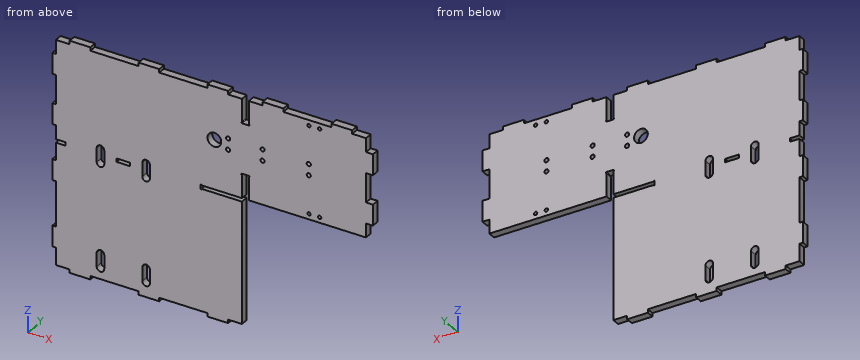
from build123d import *

# Parameters (mm, degrees)
BODY_DELETE_KEEP_START         = -69.85
BODY_DELETE_KEEP_1_OUTLINE_W   = 12.7
BODY_DELETE_KEEP_1_OUTLINE_H   = 3.175
BODY_DELETE_KEEP_1_OUTLINE_R   = 1.905
BODY_DELETE_KEEP_1_OUTLINE_R_2 = 6.35
BODY_DELETE_KEEP_1_OUTLINE_R_3 = 1.5367
BODY_DELETE_KEEP_1_DEPTH       = 6.985
SKETCH1_R                      = 0.635
CUT_EXTRUDE1_DEPTH             = 257.935529511


# Read off the part's stored shape, not the designer's step: Body-Delete/Keep 1
with BuildPart() as part:
    # Body-Delete/Keep 1 outline → Body-Delete/Keep 1 (new body)
    with BuildSketch(Plane(origin=(0, 0, 0), x_dir=(1, 0, 0), z_dir=(0, 1, 0)).offset(BODY_DELETE_KEEP_START)):
        Polygon((90.075, -13.335), (90.075, 13.335), (96.425, 13.335), (96.425, 32.385), (90.075, 32.385), (90.075, 45.085), (-17.875, 45.085), (-17.875, 22.86), (-24.225, 22.86), (-24.225, 45.085), (-62.325, 45.085), (-62.325, 48.26), (-24.225, 48.26), (-24.225, 159.385), (-36.925, 159.385), (-36.925, 162.56), (-55.975, 162.56), (-55.975, 159.385), (-100.425, 159.385), (-100.425, 162.56), (-119.475, 162.56), (-119.475, 159.385), (-163.925, 159.385), (-163.925, 162.56), (-182.975, 162.56), (-182.975, 159.385), (-195.675, 159.385), (-195.675, 143.51), (-198.85, 143.51), (-198.85, 124.46), (-195.675, 124.46), (-195.675, 83.185), (-198.85, 83.185), (-198.85, 64.135), (-195.675, 64.135), (-195.675, 48.26), (-186.785, 48.26), (-186.785, 45.085), (-195.675, 45.085), (-195.675, 32.385), (-198.85, 32.385), (-198.85, 13.335), (-195.675, 13.335), (-195.675, -13.335), (-198.85, -13.335), (-198.85, -32.385), (-195.675, -32.385), (-195.675, -45.085), (-182.975, -45.085), (-182.975, -48.26), (-163.925, -48.26), (-163.925, -45.085), (-119.475, -45.085), (-119.475, -48.26), (-100.425, -48.26), (-100.425, -45.085), (-55.975, -45.085), (-55.975, -48.26), (-36.925, -48.26), (-36.925, -45.085), (-24.225, -45.085), (-24.225, -22.86), (-17.875, -22.86), (-17.875, -45.085), (-5.175, -45.085), (-5.175, -48.26), (13.875, -48.26), (13.875, -45.085), (58.325, -45.085), (58.325, -48.26), (77.375, -48.26), (77.375, -45.085), (90.075, -45.085), (90.075, -32.385), (96.425, -32.385), (96.425, -13.335), align=None)
        with BuildLine():
            Line((-151.0668, 54.1), (-151.0668, 41.4))
            ThreePointArc((-151.0668, 41.4), (-154.5593, 37.9075), (-158.0518, 41.4))
            Line((-158.0518, 41.4), (-158.0518, 54.1))
            ThreePointArc((-158.0518, 54.1), (-154.5593, 57.5925), (-151.0668, 54.1))
        make_face(mode=Mode.SUBTRACT)
        with Locations((-133.5593, 46.6725)):
            Rectangle(BODY_DELETE_KEEP_1_OUTLINE_W, BODY_DELETE_KEEP_1_OUTLINE_H, mode=Mode.SUBTRACT)
        with BuildLine():
            Line((-109.0668, 54.1), (-109.0668, 41.4))
            ThreePointArc((-109.0668, 41.4), (-112.5593, 37.9075), (-116.0518, 41.4))
            Line((-116.0518, 41.4), (-116.0518, 54.1))
            ThreePointArc((-116.0518, 54.1), (-112.5593, 57.5925), (-109.0668, 54.1))
        make_face(mode=Mode.SUBTRACT)
        with Locations((-36.925, -5.08)):
            Circle(BODY_DELETE_KEEP_1_OUTLINE_R, mode=Mode.SUBTRACT)
        with Locations((-49.625, 0)):
            Circle(BODY_DELETE_KEEP_1_OUTLINE_R_2, mode=Mode.SUBTRACT)
        with Locations((-5.175, -5.08)):
            Circle(BODY_DELETE_KEEP_1_OUTLINE_R, mode=Mode.SUBTRACT)
        with Locations((37.5, -40.11)):
            Circle(BODY_DELETE_KEEP_1_OUTLINE_R_3, mode=Mode.SUBTRACT)
        with Locations((47.4, -40.11)):
            Circle(BODY_DELETE_KEEP_1_OUTLINE_R_3, mode=Mode.SUBTRACT)
        with Locations((37.37, -5.08)):
            Circle(BODY_DELETE_KEEP_1_OUTLINE_R, mode=Mode.SUBTRACT)
        with Locations((-36.925, 5.08)):
            Circle(BODY_DELETE_KEEP_1_OUTLINE_R, mode=Mode.SUBTRACT)
        with Locations((-5.175, 5.08)):
            Circle(BODY_DELETE_KEEP_1_OUTLINE_R, mode=Mode.SUBTRACT)
        with Locations((37.37, 5.08)):
            Circle(BODY_DELETE_KEEP_1_OUTLINE_R, mode=Mode.SUBTRACT)
        with Locations((37.5, 40.11)):
            Circle(BODY_DELETE_KEEP_1_OUTLINE_R_3, mode=Mode.SUBTRACT)
        with Locations((47.4, 40.11)):
            Circle(BODY_DELETE_KEEP_1_OUTLINE_R_3, mode=Mode.SUBTRACT)
        with BuildLine():
            Line((-158.0518, 136.4), (-158.0518, 149.1))
            ThreePointArc((-158.0518, 149.1), (-154.5593, 152.5925), (-151.0668, 149.1))
            Line((-151.0668, 149.1), (-151.0668, 136.4))
            ThreePointArc((-151.0668, 136.4), (-154.5593, 132.9075), (-158.0518, 136.4))
        make_face(mode=Mode.SUBTRACT)
        with BuildLine():
            Line((-116.0518, 136.4), (-116.0518, 149.1))
            ThreePointArc((-116.0518, 149.1), (-112.5593, 152.5925), (-109.0668, 149.1))
            Line((-109.0668, 149.1), (-109.0668, 136.4))
            ThreePointArc((-109.0668, 136.4), (-112.5593, 132.9075), (-116.0518, 136.4))
        make_face(mode=Mode.SUBTRACT)
    extrude(amount=BODY_DELETE_KEEP_1_DEPTH)

    # Sketch1 → Cut-Extrude1 (cut, through all)
    with BuildSketch(Plane(origin=(0, -62.865, 0), x_dir=(1, 0, 0), z_dir=(0, 1, 0))):
        with Locations((-61.69, 48.26)):
            Circle(SKETCH1_R)
        with Locations((-61.69, 45.085)):
            Circle(SKETCH1_R)
        with Locations((-17.875, 23.495)):
            Circle(SKETCH1_R)
        with Locations((-24.225, 23.495)):
            Circle(SKETCH1_R)
        with Locations((-17.875, -23.495)):
            Circle(SKETCH1_R)
        with Locations((-24.225, -23.495)):
            Circle(SKETCH1_R)
    extrude(amount=-CUT_EXTRUDE1_DEPTH, mode=Mode.SUBTRACT)


solid = part.part
Read the model definition and answer for the solid it produces. Units are mm, in the model's axes. Round coordinates to 2 decimals unless told otherwise and drop trailing zeros. Write each loop counter-clockwise with the first axis right and the second up, starting at its lowest first coordinate (ties: lowest second). Pieces come first, ordered by that corner, then holes.
1. Given pin 1 Ø6 at (x, z) = (-5.175, -5.08) entering from -Y; pin 2 Ø3.5 at (x, y) = (-197, -66) entering from +Z (3 decimals); pin 3 Ø1 at (y, z) = (-65.5, -47) entering from +X (3 decimals); pin 4 Ø1.6 at (y, z) = (-65.5, -161) entering from -X (3 decimals), each flat-ended and moving along its own axis, determine where each tip first touches the part or whether it passes through.
2. The part is cut by section B-B, the plane z = -115.5. Determine the outline of the cut face in (x, y) (3 decimals), then the cut area to 3 significant figures.
3. Straight lines are drawn through the part: L1, parallel to Z at x = 47.4, y = -66 (3 decimals); L2, parallel to Z at x = 37.5, y = -65.5 (3 decimals); L3, parallel to X at y = -67, z = 40.11 (3 decimals). For each, find the intervals that lie inside material, in ascending order.
4. The part is cut by section C-C, the plane y = -65.5. State how many separate pieces and enclosed holes the cut face has, then the cut area to 3 significant figures.
5. The part is cut by section A-A, the plane x = 27. Determine the outline of the cut face in (y, z) (3 decimals).
Values:
1. pin 1: stops at y = -69.85
1. pin 2: stops at z = 45.085
1. pin 3: stops at x = -62.325
1. pin 4: stops at x = -182.975
2. outline: (-195.675, -69.85) - (-24.225, -69.85) - (-24.225, -62.865) - (-195.675, -62.865) - close
2. area: 1,200 mm2
3. L1: z = -45.085 to -41.647, -38.573 to 38.573, 41.647 to 45.085
3. L2: z = -45.085 to -41.647, -38.573 to -6.981, -3.179 to 3.179, 6.981 to 38.573, 41.647 to 45.085
3. L3: x = -195.675 to -24.225, -17.875 to 35.963, 39.037 to 45.863, 48.937 to 90.075
4. separate pieces: 1
4. enclosed holes: 16
4. area: 45,100 mm2
5. outline: (-69.85, -45.085) - (-62.865, -45.085) - (-62.865, 45.085) - (-69.85, 45.085) - close
